Geometry: final body of the model. Coordinates: model frame, mm. A direction names the side the tool comes from. Give positions to 0.01 mm unless a question says otherwise; leave off trailing zeros. Order: outer loops, then holes, each group sorted by start corner. A loop starts at its lowest first (then second) coordinate and runs counter-clockwise, first axis right, second up. Notation, with made-up numbers: M 74.25,1 L 80.25,1 A15 cw 80.25,21 Z; hole C 62.5,31.5 d2. An arc over 180 degrees is marked long. One line per item, written item: value. Start each with the question number.
```python
from build123d import *

# Parameters (mm, degrees)
SKETCH1_W               = 50
SKETCH1_H               = 40
BOSS_EXTRUDE1_DEPTH     = 1
SKETCH2_R               = 1.5
BOSS_EXTRUDE2_DEPTH     = 40
SKETCH3_R               = 0.8
CUT_EXTRUDE1_DEPTH      = 49.075461516
CUT_EXTRUDE2_DEPTH      = 34.260336739
CUT_EXTRUDE2_DEPTH_BACK = 34.260336739
SKETCH4_W               = 29.985936658
SKETCH4_H               = 20
SKETCH4_W_2             = 10.666279811
SKETCH5_R               = 2.5
SKETCH5_R_2             = 1
BOSS_EXTRUDE3_DEPTH     = 3
CHAMFER1_SIZE           = 3


with BuildPart() as part:
    # Sketch1 → Boss-Extrude1 (new body)
    with BuildSketch(Plane.XY):
        Rectangle(SKETCH1_W, SKETCH1_H)
        with BuildLine():
            Line((2.2, 7.898513293), (2.2, -8.101486707))
            ThreePointArc((2.2, -8.101486707), (0, -10.301486707), (-2.2, -8.101486707))
            Line((-2.2, -8.101486707), (-2.2, 7.898513293))
            ThreePointArc((-2.2, 7.898513293), (0, 10.098513293), (2.2, 7.898513293))
        make_face(mode=Mode.SUBTRACT)
    extrude(amount=BOSS_EXTRUDE1_DEPTH)

    # Sketch2 → Boss-Extrude2 (add)
    with BuildSketch(Plane(origin=(0, 20, 0), x_dir=(1, 0, 0), z_dir=(0, 1, 0))):
        with Locations((-25, -1.5)):
            Circle(SKETCH2_R)
        with Locations((25, -1.5)):
            Circle(SKETCH2_R)
    extrude(amount=-BOSS_EXTRUDE2_DEPTH)

    # Sketch3 → Cut-Extrude1 (cut, through all)
    with BuildSketch(Plane(origin=(0, 20, 0), x_dir=(1, 0, 0), z_dir=(0, 1, 0))):
        with Locations(Location((-25, -1.5, 0), (0, 0, 270))):
            Circle(SKETCH3_R)
        with Locations(Location((25, -1.5, 0), (0, 0, 270))):
            Circle(SKETCH3_R)
    extrude(amount=-CUT_EXTRUDE1_DEPTH, mode=Mode.SUBTRACT)

    # Sketch4 → Cut-Extrude2 (cut, two sides: drawn at the far end of the back side and taken through both)
    with BuildSketch(Plane.XY.offset(1).offset(-CUT_EXTRUDE2_DEPTH_BACK)):
        with Locations((-37.492968329, 0)):
            Rectangle(SKETCH4_W, SKETCH4_H)
        with Locations((27.833139906, 0)):
            Rectangle(SKETCH4_W_2, SKETCH4_H)
    extrude(amount=CUT_EXTRUDE2_DEPTH + CUT_EXTRUDE2_DEPTH_BACK, mode=Mode.SUBTRACT)

    # Sketch5 → Boss-Extrude3 (add)
    # profile 1 of 2: a face of its own
    with BuildSketch(Plane.XY.offset(1)):
        with Locations(Location((-18.5, 0, 0), (0, 0, 180))):
            Circle(SKETCH5_R)
        with Locations((-18.5, 0)):
            Circle(SKETCH5_R_2, mode=Mode.SUBTRACT)
    # profile 2 of 2: a face of its own
    with BuildSketch(Plane.XY.offset(1)):
        with Locations(Location((18.5, 0, 0), (0, 0, 180))):
            Circle(SKETCH5_R)
        with Locations((18.5, 0)):
            Circle(SKETCH5_R_2, mode=Mode.SUBTRACT)
    extrude(amount=BOSS_EXTRUDE3_DEPTH)

    # Chamfer1
    # the kernel refuses this chamfer: 3 mm, written as the material it adds along each edge
    with BuildSketch(Plane(origin=(-18.5, 0, 1), x_dir=(-1, 0, 0), z_dir=(0, 1, 0))) as chamfer1_piece_1_section:
        Polygon((2.5 + CHAMFER1_SIZE, 0), (2.5, CHAMFER1_SIZE), (2.5, 0), align=None)
    chamfer1_piece_1 = revolve(axis=Axis((-18.5, 0, 1), (0, 0, 1)), mode=Mode.PRIVATE)
    chamfer1_piece_1 = split(chamfer1_piece_1, bisect_by=Plane(origin=(-22.5, 0, 2.424420983), z_dir=(1, 0, 0)), keep=Keep.TOP, mode=Mode.PRIVATE)
    chamfer1_piece_1 = split(chamfer1_piece_1, bisect_by=Plane(origin=(-14.490726203, 0, 4), z_dir=(0, 0, -1)), keep=Keep.TOP, mode=Mode.PRIVATE)
    add(chamfer1_piece_1)
    with BuildSketch(Plane(origin=(18.5, 0, 1), x_dir=(-1, 0, 0), z_dir=(0, 1, 0))) as chamfer1_piece_2_section:
        Polygon((2.5 + CHAMFER1_SIZE, 0), (2.5, CHAMFER1_SIZE), (2.5, 0), align=None)
    chamfer1_piece_2 = revolve(axis=Axis((18.5, 0, 1), (0, 0, 1)), mode=Mode.PRIVATE)
    chamfer1_piece_2 = split(chamfer1_piece_2, bisect_by=Plane(origin=(22.5, -4.362653262, 1.396136714), z_dir=(-1, 0, 0)), keep=Keep.TOP, mode=Mode.PRIVATE)
    chamfer1_piece_2 = split(chamfer1_piece_2, bisect_by=Plane(origin=(15.981220965, -4.362653262, 4), z_dir=(0, 0, -1)), keep=Keep.TOP, mode=Mode.PRIVATE)
    add(chamfer1_piece_2)


solid = part.part
```
Q1. Section query B-B on y = 0. Return loops of the section in (x, z).
Q2. Set-up query: faces 1 (the face through (-19, 0, 1)), 2 (the face through (0, 10.1, 0.5)), 3 (the face through (24, 10, 1)), 4 (the face through (-22.5, 0, 1)). Return all of +Z, -Z, +X, -X, +Y, -Y with unobstructed straight access to the full face (end or side cutting, diameter ignored); none if empty.
Q3. Section query A-A on x = 0. Return loops of the section in (y, z), and give its area (3 significant figures).
Q4. Ray query, line 1 along X through (y, z) = (12.5, 1.5); line 2 along Y through (x, z) = (-23.5, 0.65); line 3 along Z through (x, y) = (-17, -16.5). Return the intervals inside material, ascending. Write a range as [from, to].
Q5. Contact query for flat-ended pins moving along their axis: pin 1 (0.8 mm diameter, centred on y = 3.5, z = 0.5, fed in from -X); pin 2 (4 mm diameter, centred on x = 7.5, y = -9, fed in from +Z); pin 3 (1.2 mm diameter, centred on y = 2, z = 1.5, fed in from +X). Output: stop coordinate, or through.
Q6. Section query C-C on y = -11. Return loops of the section in (x, z).
Q7. Section query D-D on z = 1.6. Give the number of separate pieces and of enclosed holes in the cut face, and give its area (3 significant figures).
Q8. Mould query, pull axis X, two halves, no side actions, for faces 5 (the face through (22.5, 0, 1)), 6 (the face through (-24, 10, 1)), 7 (the face through (-15.857, -0.116, 3.854)). Classes: +X half, -X half, draft (parallel to the pull), parting line (faces both ways), or undercut.
Results below:
1. outline: M -22.5,0 L -2.2,0 L -2.2,1 L -13,1 L -16,4 L -17.5,4 L -17.5,1 L -19.5,1 L -19.5,4 L -21,4 L -22.5,2.5 Z; M 2.2,0 L 22.5,0 L 22.5,2.5 L 21,4 L 19.5,4 L 19.5,1 L 17.5,1 L 17.5,4 L 16,4 L 13,1 L 2.2,1 Z
2. face 1: +Z
2. face 2: +Z, -Z
2. face 3: +Z, -Z, +X
2. face 4: +Z, -Z, -X
3. outline: M -20,0 L -10.3,0 L -10.3,1 L -20,1 Z; M 10.1,0 L 20,0 L 20,1 L 10.1,1 Z
3. area: 19.6 mm2
4. line 1: [-26.5, -25.8], [-24.2, -23.5], [23.5, 24.2], [25.8, 26.5]
4. line 2: [-20, -10], [10, 20]
4. line 3: [0, 1]
5. pin 1: x = -22.5
5. pin 2: z = 1
5. pin 3: x = 22.5
6. outline: M -25,0 L 25,0 A1.5 ccw long 23.59,1 L -23.59,1 A1.5 ccw long Z; hole C -25,1.5 d1.6; hole C 25,1.5 d1.6
7. separate pieces: 10
7. enclosed holes: 2
7. area: 194 mm2
8. face 5: +X half
8. face 6: draft
8. face 7: undercut
